Model file for the job. Use its own axes, mm. A direction names the side the tool comes from. Give positions to 0.01 mm unless a question says otherwise; leave off trailing zeros. Loops run counter-clockwise (first coordinate to the right, second up) from the corner with the lowest first, then second, coordinate; pieces in that order, holes last. Notation, with made-up numbers: M -2.75,3.25 L 23.25,3.25 A26 cw 23.25,39.25 Z; hole C -21,-33.5 d2. An arc over 180 degrees is marked long. Use CSV: the item, a comma, the result in double quotes. Start each with the question number.
(1) Flat gauge pins, fed straight in: P1, Ø3, axis at x = -5.5, y = -2.5, coming from the +Z side; P2, Ø4.5, axis at y = 0.08, z = 55.47, coming from the +X side; P3, Ø1.5, axis at y = 0, z = 28.5, coming from the +X side; P4, Ø1.5, axis at x = 0, z = 27, coming from the +Y side. Where does each tip first touch, or does it go through?
(2) Two-plate mould, pull along Z, no slides. Class faces 5 (the face through (11, 0, -16)), 6 (the face through (1, 5, 7)), 7 (the face through (-10, 0, -5)): pulls with the +Z half, pulls with the -Z half, needs draft (parallel to the pull), parting line crosses it, or undercut.
(3) Tool access for faces 1 (the face through (-12, 0, -4)), 2 (the face through (0, 1.5, 30)), 3 (the face through (-0.1, -0.4, -10.1)), 4 (the face through (-2.5, 0, 30)): list every direction of +Z, -Z, +X, -X, +Y, -Y with a clear straight run to the whole face (end or side of a thin tool).
(4) Slice it at B-B on y = -0.75. List the corners of the cut face in (x, z), and give its area (3 significant figures).
(5) Slice it at C-C on x = 9.25. List the corners of the cut face in (y, z).
(6) Slice it at A-A on z = 3.5. List the corners of the cut face in (x, y).
(7) Slice it at D-D on z = 35. List the corners of the cut face in (x, y), and give its area (3 significant figures).
(8) Wall check: line 1 along Z through (x, y) = (4.5, 0); line 2 along X through (y, z) = (-3.5, -4); line 3 along Z through (x, y) = (-5, 0.75). Give the ranges that are in metal, low to high. Write a range as from..to.
Solid Edge part; units mm, degrees
sketch "Sketch1" plane through (0, 0, 0) normal (0, -1, 0) x (1, 0, 0)
  line L0 (-12, 9) -> (12, 9)
  line L1 (12, 9) -> (12, -16)
  line L2 (10, -16) -> (12, -16)
  line L3 (10, -16) -> (10, 6)
  line L4 (10, 6) -> (-10, 6)
  line L5 (-10, 6) -> (-10, -16)
  line L6 (-12, -16) -> (-10, -16)
  line L7 (-12, -16) -> (-12, 9)
extrude "Protrusion1" add sketch "Sketch1" along normal mid plane 10
sketch "Sketch2" plane through (-10, 0, -5) normal (1, 0, 0) x (0, 1, 0)
  circle A0 centre (0, -7.0612) radius 2
extrude "ExtrudedProtrusion_5" add sketch "Sketch2" along normal blind 20
sketch "Sketch3" plane through (0, 0, 9) normal (0, 0, 1) x (1, 0, 0)
  line L0 (2.5, -1.5) -> (2.5, 1.5)
  line L1 (2.5, 1.5) -> (-2.5, 1.5)
  line L2 (-2.5, 1.5) -> (-2.5, -1.5)
  line L3 (-2.5, -1.5) -> (2.5, -1.5)
extrude "ExtrudedProtrusion_6" add sketch "Sketch3" along normal blind 50
sketch "Sketch4" plane through (-2.5, 0, 34) normal (-1, 0, 0) x (0, 0, 1)
  circle A0 centre (21.4608, 0.0773) radius 3.5
extrude "ExtrudedProtrusion_8" add sketch "Sketch4" along normal blind 12 and the other way blind 17
sketch "Sketch5" plane through (-16.5, 0.0773, 55.4608) normal (-1, 0, 0) x (0, 0, 1)
  circle A0 centre (0.0121, 0) radius 2.5
extrude "ExtrudedCutout_1" cut sketch "Sketch5" against normal blind 62.1313
Reply:
1,P1,"stops at z = 58.79"
1,P2,"passes through"
1,P3,"stops at x = 2.5"
1,P4,"stops at y = 1.5"
2,face 5,"pulls with the -Z half"
2,face 6,"needs draft"
2,face 7,"undercut"
3,face 1,"-Z, -X, +Y, -Y"
3,face 2,"+X, -X, +Y"
3,face 3,"none"
3,face 4,"-X, +Y, -Y"
4,outline,"M -14.5,52.06 L -2.5,52.06 L -2.5,9 L -12,9 L -12,-16 L -10,-16 L -10,-13.92 L 10,-13.92 L 10,-16 L 12,-16 L 12,9 L 2.5,9 L 2.5,52.06 L 14.5,52.06 L 14.5,53.11 L -14.5,53.11 Z; M -14.5,57.83 L 14.5,57.83 L 14.5,58.86 L 2.5,58.86 L 2.5,59 L -2.5,59 L -2.5,58.86 L -14.5,58.86 Z; hole M -10,-10.21 L 10,-10.21 L 10,6 L -10,6 Z"
4,area,"511 mm^2"
5,outline,"M -5,6 L 5,6 L 5,9 L -5,9 Z; C 0.08,55.46 d7; C 0,-12.06 d4; hole C 0.08,55.47 d5"
6,outline,"M -12,-5 L -10,-5 L -10,5 L -12,5 Z; M 10,-5 L 12,-5 L 12,5 L 10,5 Z"
7,outline,"M -2.5,-1.5 L 2.5,-1.5 L 2.5,1.5 L -2.5,1.5 Z"
7,area,"15.0 mm^2"
8,line 1,"z = -14.06..-10.06, 6..9, 51.96..52.97, 57.97..58.96"
8,line 2,"x = -12..-10, 10..12"
8,line 3,"z = -13.92..-10.21, 6..9, 52.03..53.07, 57.88..58.9"
